Part model, mm, in its own coordinate system. A direction names the side the tool comes from. Round coordinates to 2 decimals unless told otherwise and drop trailing zeros. Loops run counter-clockwise (first coordinate to the right, second up) from the corner with the lowest first, then second, coordinate; pieces in that order, holes last.
(1) Cut at B-B on y = 17.5. List the corners of the cut face in (x, z), then the cut area to 3 significant figures.
(2) Cut at A-A on z = 22.5. List the corners of the cut face in (x, y), then the cut area to 3 significant figures.
(3) Flat gauge pins, fed straight in: pin 1 (3.5 mm diameter, centred on y = -26.5, z = -5.5, fed in from +X); pin 2 (3 mm diameter, centred on x = -24.5, y = 1, fed in from +Z); pin 3 (4.5 mm diameter, centred on x = -26, y = -26, fed in from +Z). Where does each tip first touch, or does it go through?
(4) Cut at D-D on z = 10.5. Count the separate pieces of the cut face and the enclosed holes in it, then the cut area to 3 significant figures.
(5) Tool access for faces 4 (the face through (-30, 31, 29)), 5 (the face through (0, 34.747, 0)): list every direction of +Z, -Z, +X, -X, +Y, -Y with a clear straight run to the whole face (end or side of a thin tool).
(6) Probe probe 1 along Y at (x, z) = (7.5, -21); probe 2 along X at (y, z) = (21, -20). List the from-to ranges inside material, lowest first.
(7) Mould opens along Y. For faces 1 (the face through (31, 30, 29)), 2 (the face through (-34, 10, 29.21)), 3 (the face through (0, -34.747, 0)) say: +Y half, -Y half, draft (parallel to the pull), parting line (faces both ways), or undercut.
from build123d import *

# Parameters (mm, degrees)
BOSS_EXTRUDE1_DEPTH          = 29.21
SHELL1_T                     = -2.54
FILLET1_R                    = 6.35
BOSS_EXTRUDE2_DEPTH          = 38.1
SKETCH3_R                    = 2.8067
CUT_EXTRUDE1_DEPTH           = 4.7
CUT_EXTRUDE1_DRAFT           = -8
CUT_EXTRUDE1_PROFILE_2_DEPTH = 4.7
CUT_EXTRUDE1_PROFILE_2_DRAFT = -8
CUT_EXTRUDE1_PROFILE_3_DEPTH = 4.7
CUT_EXTRUDE1_PROFILE_3_DRAFT = -8
CUT_EXTRUDE1_PROFILE_4_DEPTH = 4.7
CUT_EXTRUDE1_PROFILE_4_DRAFT = -8
SKETCH5_W                    = 45.253999916
SKETCH5_H                    = 45.253999916
CUT_EXTRUDE5_DEPTH           = 38.1
SKETCH6_OUTSIDE_W            = 88.184
SKETCH6_OUTSIDE_H            = 88.184
CUT_EXTRUDE6_DEPTH           = 1.3208
BOSS_EXTRUDE3_START          = -2.54
BOSS_EXTRUDE3_DEPTH          = 57.0992
BOSS_EXTRUDE7_START          = -57.0992
BOSS_EXTRUDE7_DEPTH          = 58.42


with BuildPart() as part:
    # Sketch1 → Boss-Extrude1 (new, symmetric)
    with BuildSketch(Plane.XY):
        Polygon((-32.258, -32.258), (-32.258, -11.938), (-32.258, 11.938), (-32.258, 32.258), (32.258, 32.258), (32.258, -32.258), align=None)
    extrude(amount=BOSS_EXTRUDE1_DEPTH, both=True)

    # Shell1
    shell1_openings = [part.faces().sort_by_distance(p)[0] for p in [
        (0, 0, 29.21),
    ]]
    offset(amount=SHELL1_T, openings=shell1_openings, kind=Kind.INTERSECTION)

    # Fillet1
    fillet1_edges = [part.edges().sort_by_distance(p)[0] for p in [
        (-32.258, -32.258, 0),
        (-32.258, 32.258, 0),
        (32.258, 32.258, 0),
        (32.258, -32.258, 0),
        (-29.718, -29.718, 1.27),
        (29.718, -29.718, 1.27),
        (29.718, 29.718, 1.27),
        (-29.718, 29.718, 1.27),
    ]]
    fillet(fillet1_edges, radius=FILLET1_R)

    # Sketch2 → Boss-Extrude2 (add)
    with BuildSketch(Plane.XY.offset(-26.67)):
        with BuildLine():
            Line((-20.828, -20.828), (-29.718, -20.828))
            Line((-29.718, -20.828), (-29.718, -23.368))
            ThreePointArc((-29.718, -23.368), (-27.858128061, -27.858128061), (-23.368, -29.718))
            Line((-23.368, -29.718), (-20.828, -29.718))
            Line((-20.828, -29.718), (-20.828, -20.828))
        make_face()
        with BuildLine():
            ThreePointArc((-29.718, 23.368), (-27.858128061, 27.858128061), (-23.368, 29.718))
            Line((-23.368, 29.718), (-20.828, 29.718))
            Line((-20.828, 29.718), (-20.828, 20.828))
            Line((-20.828, 20.828), (-29.718, 20.828))
            Line((-29.718, 20.828), (-29.718, 23.368))
        make_face()
        with BuildLine():
            ThreePointArc((29.718, 23.368), (27.858128061, 27.858128061), (23.368, 29.718))
            Line((23.368, 29.718), (20.828, 29.718))
            Line((20.828, 29.718), (20.828, 20.828))
            Line((20.828, 20.828), (29.718, 20.828))
            Line((29.718, 20.828), (29.718, 23.368))
        make_face()
        with BuildLine():
            ThreePointArc((23.368, -29.718), (27.858128061, -27.858128061), (29.718, -23.368))
            Line((29.718, -23.368), (29.718, -20.828))
            Line((29.718, -20.828), (20.828, -20.828))
            Line((20.828, -20.828), (20.828, -29.718))
            Line((20.828, -29.718), (23.368, -29.718))
        make_face()
    extrude(amount=BOSS_EXTRUDE2_DEPTH)


with BuildPart() as cut_extrude1_tool:
    # Sketch3 → Cut-Extrude1 (with draft: the straight prism first)
    with BuildSketch(Plane.XY.offset(11.43)):
        with Locations((-25.4, -25.4)):
            Circle(SKETCH3_R)
    extrude(amount=-CUT_EXTRUDE1_DEPTH)
    # Cut-Extrude1: the draft: its side faces are tilted about the plane it starts from
    cut_extrude1_sides = [cut_extrude1_tool.faces().sort_by_distance(p)[0] for p in [
        (-28.2067, -25.4, 9.08),
    ]]
    draft(cut_extrude1_sides, Plane.XY.offset(11.43), CUT_EXTRUDE1_DRAFT)


with BuildPart() as part_1:
    add(part.part)

    # Cut-Extrude1: cut by cut_extrude1_tool
    add(cut_extrude1_tool.part, mode=Mode.SUBTRACT)


with BuildPart() as cut_extrude1_profile_2_tool:
    # Sketch3 → Cut-Extrude1 profile 2 (with draft: the straight prism first)
    with BuildSketch(Plane.XY.offset(11.43)):
        with Locations((-25.4, 25.4)):
            Circle(SKETCH3_R)
    extrude(amount=-CUT_EXTRUDE1_PROFILE_2_DEPTH)
    # Cut-Extrude1 profile 2: the draft: its side faces are tilted about the plane it starts from
    cut_extrude1_profile_2_sides = [cut_extrude1_profile_2_tool.faces().sort_by_distance(p)[0] for p in [
        (-28.2067, 25.4, 9.08),
    ]]
    draft(cut_extrude1_profile_2_sides, Plane.XY.offset(11.43), CUT_EXTRUDE1_PROFILE_2_DRAFT)


with BuildPart() as part_2:
    add(part_1.part)

    # Cut-Extrude1 profile 2: cut by cut_extrude1_profile_2_tool
    add(cut_extrude1_profile_2_tool.part, mode=Mode.SUBTRACT)


with BuildPart() as cut_extrude1_profile_3_tool:
    # Sketch3 → Cut-Extrude1 profile 3 (with draft: the straight prism first)
    with BuildSketch(Plane.XY.offset(11.43)):
        with Locations((25.4, 25.4)):
            Circle(SKETCH3_R)
    extrude(amount=-CUT_EXTRUDE1_PROFILE_3_DEPTH)
    # Cut-Extrude1 profile 3: the draft: its side faces are tilted about the plane it starts from
    cut_extrude1_profile_3_sides = [cut_extrude1_profile_3_tool.faces().sort_by_distance(p)[0] for p in [
        (22.5933, 25.4, 9.08),
    ]]
    draft(cut_extrude1_profile_3_sides, Plane.XY.offset(11.43), CUT_EXTRUDE1_PROFILE_3_DRAFT)


with BuildPart() as part_3:
    add(part_2.part)

    # Cut-Extrude1 profile 3: cut by cut_extrude1_profile_3_tool
    add(cut_extrude1_profile_3_tool.part, mode=Mode.SUBTRACT)


with BuildPart() as cut_extrude1_profile_4_tool:
    # Sketch3 → Cut-Extrude1 profile 4 (with draft: the straight prism first)
    with BuildSketch(Plane.XY.offset(11.43)):
        with Locations((25.4, -25.4)):
            Circle(SKETCH3_R)
    extrude(amount=-CUT_EXTRUDE1_PROFILE_4_DEPTH)
    # Cut-Extrude1 profile 4: the draft: its side faces are tilted about the plane it starts from
    cut_extrude1_profile_4_sides = [cut_extrude1_profile_4_tool.faces().sort_by_distance(p)[0] for p in [
        (22.5933, -25.4, 9.08),
    ]]
    draft(cut_extrude1_profile_4_sides, Plane.XY.offset(11.43), CUT_EXTRUDE1_PROFILE_4_DRAFT)


with BuildPart() as part_4:
    add(part_3.part)

    # Cut-Extrude1 profile 4: cut by cut_extrude1_profile_4_tool
    add(cut_extrude1_profile_4_tool.part, mode=Mode.SUBTRACT)

    # Sketch5 → Cut-Extrude5 (cut)
    with BuildSketch(Plane.XY.offset(11.43)):
        Rectangle(SKETCH5_W, SKETCH5_H)
    extrude(amount=-CUT_EXTRUDE5_DEPTH, mode=Mode.SUBTRACT)

    # Sketch6 outside → Cut-Extrude6 (cut)
    # profile 1 of 2: a face of its own
    with BuildSketch(Plane.XY.offset(29.21)):
        Rectangle(SKETCH6_OUTSIDE_W, SKETCH6_OUTSIDE_H)
        with BuildLine():
            Line((23.368, 30.988), (20.828, 30.988))
            Line((20.828, 30.988), (-20.828, 30.988))
            Line((-20.828, 30.988), (-23.368, 30.988))
            ThreePointArc((-23.368, 30.988), (-28.756153673, 28.756153673), (-30.988, 23.368))
            Line((-30.988, 23.368), (-30.988, -23.368))
            ThreePointArc((-30.988, -23.368), (-28.756153673, -28.756153673), (-23.368, -30.988))
            Line((-23.368, -30.988), (-20.828, -30.988))
            Line((-20.828, -30.988), (20.828, -30.988))
            Line((20.828, -30.988), (23.368, -30.988))
            ThreePointArc((23.368, -30.988), (28.756153673, -28.756153673), (30.988, -23.368))
            Line((30.988, -23.368), (30.988, 23.368))
            ThreePointArc((30.988, 23.368), (28.756153673, 28.756153673), (23.368, 30.988))
        make_face(mode=Mode.SUBTRACT)
    # profile 2 of 2: a face of its own
    with BuildSketch(Plane.XY.offset(29.21)):
        with BuildLine():
            Line((23.368, 29.718), (20.828, 29.718))
            Line((20.828, 29.718), (-20.828, 29.718))
            Line((-20.828, 29.718), (-23.368, 29.718))
            ThreePointArc((-23.368, 29.718), (-27.858128061, 27.858128061), (-29.718, 23.368))
            Line((-29.718, 23.368), (-29.718, -23.368))
            ThreePointArc((-29.718, -23.368), (-27.858128061, -27.858128061), (-23.368, -29.718))
            Line((-23.368, -29.718), (-20.828, -29.718))
            Line((-20.828, -29.718), (20.828, -29.718))
            Line((20.828, -29.718), (23.368, -29.718))
            ThreePointArc((23.368, -29.718), (27.858128061, -27.858128061), (29.718, -23.368))
            Line((29.718, -23.368), (29.718, 23.368))
            ThreePointArc((29.718, 23.368), (27.858128061, 27.858128061), (23.368, 29.718))
        make_face()
    extrude(amount=-CUT_EXTRUDE6_DEPTH, mode=Mode.SUBTRACT)

    # Sketch7 → Boss-Extrude3 (add)
    with BuildSketch(Plane.XY.offset(-26.67).offset(BOSS_EXTRUDE3_START)):
        with BuildLine():
            Line((33.4772, -23.368), (33.4772, 23.368))
            ThreePointArc((33.4772, 23.368), (30.516283872, 30.516283872), (23.368, 33.4772))
            Line((23.368, 33.4772), (-23.368, 33.4772))
            ThreePointArc((-23.368, 33.4772), (-30.516283872, 30.516283872), (-33.4772, 23.368))
            Line((-33.4772, 23.368), (-33.4772, -23.368))
            ThreePointArc((-33.4772, -23.368), (-30.516283872, -30.516283872), (-23.368, -33.4772))
            Line((-23.368, -33.4772), (23.368, -33.4772))
            ThreePointArc((23.368, -33.4772), (30.516283872, -30.516283872), (33.4772, -23.368))
        make_face()
        with BuildLine():
            Line((23.368, 32.2072), (-23.368, 32.2072))
            ThreePointArc((-23.368, 32.2072), (-29.61825826, 29.61825826), (-32.2072, 23.368))
            Line((-32.2072, 23.368), (-32.2072, -23.368))
            ThreePointArc((-32.2072, -23.368), (-29.61825826, -29.61825826), (-23.368, -32.2072))
            Line((-23.368, -32.2072), (23.368, -32.2072))
            ThreePointArc((23.368, -32.2072), (29.61825826, -29.61825826), (32.2072, -23.368))
            Line((32.2072, -23.368), (32.2072, 23.368))
            ThreePointArc((32.2072, 23.368), (29.61825826, 29.61825826), (23.368, 32.2072))
        make_face(mode=Mode.SUBTRACT)
    extrude(amount=BOSS_EXTRUDE3_DEPTH)

    # Sketch9 → Boss-Extrude7 (add)
    with BuildSketch(Plane.XY.offset(27.8892).offset(BOSS_EXTRUDE7_START)):
        with BuildLine():
            Line((34.7472, -23.368), (34.7472, 23.368))
            ThreePointArc((34.7472, 23.368), (31.414309484, 31.414309484), (23.368, 34.7472))
            Line((23.368, 34.7472), (-23.368, 34.7472))
            ThreePointArc((-23.368, 34.7472), (-31.414309484, 31.414309484), (-34.7472, 23.368))
            Line((-34.7472, 23.368), (-34.7472, -23.368))
            ThreePointArc((-34.7472, -23.368), (-31.414309484, -31.414309484), (-23.368, -34.7472))
            Line((-23.368, -34.7472), (23.368, -34.7472))
            ThreePointArc((23.368, -34.7472), (31.414309484, -31.414309484), (34.7472, -23.368))
        make_face()
        with BuildLine():
            Line((23.368, 33.4772), (-23.368, 33.4772))
            ThreePointArc((-23.368, 33.4772), (-30.516283872, 30.516283872), (-33.4772, 23.368))
            Line((-33.4772, 23.368), (-33.4772, -23.368))
            ThreePointArc((-33.4772, -23.368), (-30.516283872, -30.516283872), (-23.368, -33.4772))
            Line((-23.368, -33.4772), (23.368, -33.4772))
            ThreePointArc((23.368, -33.4772), (30.516283872, -30.516283872), (33.4772, -23.368))
            Line((33.4772, -23.368), (33.4772, 23.368))
            ThreePointArc((33.4772, 23.368), (30.516283872, 30.516283872), (23.368, 33.4772))
        make_face(mode=Mode.SUBTRACT)
    extrude(amount=BOSS_EXTRUDE7_DEPTH)


solid = part_4.part
Final values:
1. outline: (-34.75, -29.21) - (34.75, -29.21) - (34.75, 29.21) - (33.48, 29.21) - (33.48, 27.89) - (30.99, 27.89) - (30.99, 29.21) - (29.72, 29.21) - (29.72, -26.67) - (-29.72, -26.67) - (-29.72, 29.21) - (-30.99, 29.21) - (-30.99, 27.89) - (-33.48, 27.89) - (-33.48, 29.21) - (-34.75, 29.21) - close
1. area: 732 mm2
2. outline: (-34.75, -23.37) arc R11.38 ccw to (-23.37, -34.75) - (23.37, -34.75) arc R11.38 ccw to (34.75, -23.37) - (34.75, 23.37) arc R11.38 ccw to (23.37, 34.75) - (-23.37, 34.75) arc R11.38 ccw to (-34.75, 23.37) - close; hole (-29.72, -23.37) arc R6.35 ccw to (-23.37, -29.72) - (23.37, -29.72) arc R6.35 ccw to (29.72, -23.37) - (29.72, 23.37) arc R6.35 ccw to (23.37, 29.72) - (-23.37, 29.72) arc R6.35 ccw to (-29.72, 23.37) - close
2. area: 1,220 mm2
3. pin 1: stops at x = 34.66
3. pin 2: stops at z = -26.67
3. pin 3: stops at z = 11.43
4. separate pieces: 1
4. enclosed holes: 5
4. area: 1,400 mm2
5. face 4: +Z
5. face 5: +Z, -Z, +X, -X, +Y
6. probe 1: y = -34.75 to -29.72, 29.72 to 34.75
6. probe 2: x = -34.75 to -22.63, 22.63 to 34.75
7. face 1: undercut
7. face 2: draft
7. face 3: -Y half
